For this review, take the finished solid that the model builds, in its own axes (mm). A direction names the side the tool comes from. Give positions to 0.01 mm unless a question says otherwise; leave off trailing zeros. Write each loop counter-clockwise with the first axis right and the second up, starting at its lowest first coordinate (ties: lowest second). Pieces come first, ordered by that corner, then holes.
Q1. Mouldability with a two-part tool opening along Y and no side actions: class faces 1 (the cylindrical face through (0.507, 1.717, 0.541)), 2 (the flat face through (-2, 0, -0.75)), 3 (the flat face through (5, 0, 0)) as released by +Y, released by -Y, zero draft, split by the parting line, or undercut.
Q2. We need section B-B (x = 0.5). Write out the cut boundary in (y, z).
Q3. We need section C-C (x = 4.5). Write out the cut boundary in (y, z), then the cut area to 3 significant figures.
Q4. We need section A-A (x = -2). Write out the cut boundary in (y, z).
Q5. For line 1 (X direction, y = 1.3, z = -1); line 2 (Z direction, x = -1.25, y = 0.6); line 3 (Z direction, x = -1.5, y = 0.1), list the stretches that pass through material, from the lowest coordinate up.
Q6. Machinability: for faces 4 (the cylindrical face through (2.87, -1.5, 0.07)), 5 (the flat face through (-2.42, 0, -1)), 6 (the cylindrical face through (-1.11, -1.5, 0.07)), which of the approach directions +Z, -Z, +X, -X, +Y, -Y give a long, thin tool a straight path to every point of the face, cutting with its end or side? Answer none if there is none.
Autodesk Inventor part; units mm, degrees
ref_plane "shaft_to_bearing_XY" through (0, 0, 0) normal (1, 0, 0) x (0, 0, -1)
ref_plane "shaft_to_bearing_YZ" through (0, 0, 0) normal (0, 0, -1) x (0, 1, 0)
ref_plane "shaft_to_bearing_ZX" through (0, 0, 0) normal (0, 1, 0) x (1, 0, 0)
sketch "Sketch_1" plane through (0, 0, 0) normal (0, 0, 1) x (1, 0, 0)
  line L0 (1, 0) -> (-2.42, 0)
  line L1 (-2.42, 0) -> (-2.42, 1.3)
  line L2 (-2.42, 1.3) -> (-2.22, 1.5)
  line L3 (-2.22, 1.5) -> (-0.04, 1.5)
  arc A0 (-0.04, 1.5) -> (0, 1.54) centre (-0.04, 1.54) ccw
  line L4 (0, 1.54) -> (0, 1.8)
  line L5 (0, 1.8) -> (1, 1.8)
  line L6 (1, 1.8) -> (1, 0)
  line L7 (1, 0) -> (-2.42, 0)
revolve "Revolution1" add sketch "Sketch_1" angle 360 about axis through (1, 0, 0) along (1, 0, 0)
sketch "Sketch_5" plane through (0, 0, 0) normal (0, 0, 1) x (1, 0, 0)
  line L0 (5, 0) -> (1, 0)
  line L1 (1, 0) -> (1, 1.5)
  line L2 (1, 1.5) -> (4.6935, 1.5)
  line L3 (4.6935, 1.5) -> (5, 1.1935)
  line L4 (5, 1.1935) -> (5, 0)
  line L5 (5, 0) -> (1, 0)
revolve "Revolution2" add sketch "Sketch_5" angle 360 about axis through (5, 0, 0) along (1, 0, 0)
thread "Thread1"
sketch "Sketch_2" plane through (-2.42, 0, 0) normal (1, 0, 0) x (0, 0, -1)
  line L0 (-0.75, -0.433) -> (0, -0.866)
  line L1 (0, -0.866) -> (0.75, -0.433)
  line L2 (0.75, -0.433) -> (0.75, 0.433)
  line L3 (0.75, 0.433) -> (0, 0.866)
  line L4 (0, 0.866) -> (-0.75, 0.433)
  line L5 (-0.75, 0.433) -> (-0.75, -0.433)
extrude "Extrusion1" cut sketch "Sketch_2" along normal blind 1.5
sketch "Sketch_3" plane through (0, 0, 0) normal (0, 0, 1) x (1, 0, 0)
  line L0 (-0.487, 0) -> (-0.92, 0)
  line L1 (-0.92, 0) -> (-0.92, 0.75)
  line L2 (-0.92, 0.75) -> (-0.487, 0)
  line L3 (-0.487, 0) -> (-0.92, 0)
revolve "Revolution3" cut sketch "Sketch_3" angle 360 about axis through (-0.487, 0, 0) along (1, 0, 0)
ref_plane "shaft_to_bearing_XY" through (0, 0, 0) normal (1, 0, 0) x (0, 0, -1)
ref_plane "shaft_to_bearing_YZ" through (0, 0, 0) normal (0, 0, -1) x (0, 1, 0)
ref_plane "shaft_to_bearing_ZX" through (0, 0, 0) normal (0, 1, 0) x (1, 0, 0)
properties part number "NTBG6-4_a"
Computed:
1. face 1: split by the parting line
1. face 2: undercut
1. face 3: zero draft
2. outline: circle Ø3.6 at (0, 0)
3. outline: circle Ø3 at (0, 0)
3. area: 7.07 mm2
4. outline: circle Ø3 at (0, 0); hole (-0.87, 0) - (-0.43, -0.75) - (0.43, -0.75) - (0.87, 0) - (0.43, 0.75) - (-0.43, 0.75) - close
5. line 1: x = 0 to 1
5. line 2: z = -1.37 to -0.46, 0.46 to 1.37
5. line 3: z = -1.5 to -0.75, 0.75 to 1.5
6. face 4: +X
6. face 5: +Z, -Z, -X, +Y, -Y
6. face 6: -X
